from build123d import *

# Parameters (mm, degrees)
SKETCH1_W           = 82.6
SKETCH1_H           = 98
BOSS_EXTRUDE1_DEPTH = 1.2
SKETCH2_R           = 1.65
CUT_EXTRUDE1_DEPTH  = 129.172539961
SKETCH3_R           = 35
BOSS_EXTRUDE2_DEPTH = 8
SKETCH4_R           = 37
BOSS_EXTRUDE3_DEPTH = 1
SKETCH5_R           = 32
CUT_EXTRUDE2_DEPTH  = 129.572158728
CHAMFER1_SIZE       = 1


with BuildPart() as part:
    # Sketch1 → Boss-Extrude1 (new body)
    with BuildSketch(Plane.YZ):
        with Locations((41.3, 49)):
            Rectangle(SKETCH1_W, SKETCH1_H)
    extrude(amount=BOSS_EXTRUDE1_DEPTH)

    # Sketch2 → Cut-Extrude1 (cut, through all)
    with BuildSketch(Plane.YZ.offset(1.2)):
        with Locations(Location((3.2, 94.8, 0), (0, 0, 270))):
            Circle(SKETCH2_R)
        with Locations(Location((79.4, 94.8, 0), (0, 0, 270))):
            Circle(SKETCH2_R)
        with Locations(Location((3.2, 3.2, 0), (0, 0, 270))):
            Circle(SKETCH2_R)
        with Locations(Location((79.4, 3.2, 0), (0, 0, 270))):
            Circle(SKETCH2_R)
    extrude(amount=-CUT_EXTRUDE1_DEPTH, mode=Mode.SUBTRACT)

    # Sketch3 → Boss-Extrude2 (add)
    with BuildSketch(Plane.YZ.offset(1.2)):
        with Locations(Location((41.3, 49, 0), (0, 0, 270))):
            Circle(SKETCH3_R)
    extrude(amount=BOSS_EXTRUDE2_DEPTH)

    # Sketch4 → Boss-Extrude3 (add)
    with BuildSketch(Plane.YZ.offset(9.2)):
        with Locations(Location((41.3, 49, 0), (0, 0, 270))):
            Circle(SKETCH4_R)
    extrude(amount=BOSS_EXTRUDE3_DEPTH)

    # Sketch5 → Cut-Extrude2 (cut, through all)
    with BuildSketch(Plane.YZ.offset(10.2)):
        with Locations(Location((41.3, 49, 0), (0, 0, 270))):
            Circle(SKETCH5_R)
    extrude(amount=-CUT_EXTRUDE2_DEPTH, mode=Mode.SUBTRACT)

    # Chamfer1
    chamfer1_edges = [part.edges().sort_by_distance(p)[0] for p in [
        (0, 79.4, 96.45),
        (0, 3.2, 4.85),
        (0, 79.4, 4.85),
        (0, 3.2, 96.45),
        (0, 41.3, 81),
        (10.2, 41.3, 81),
    ]]
    chamfer(chamfer1_edges, length=CHAMFER1_SIZE)


solid = part.part
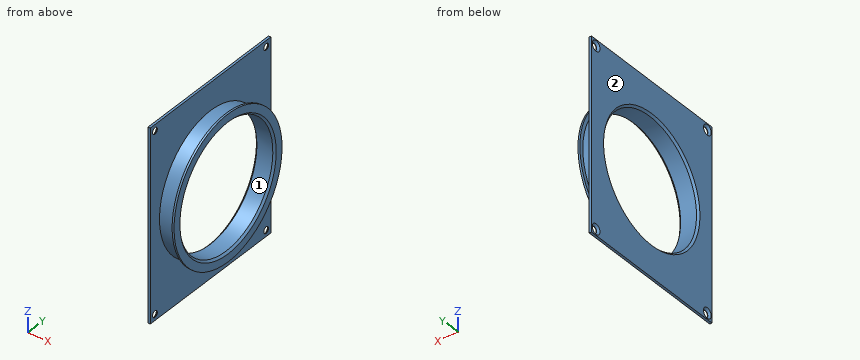
Source: CAD feature listing. Evaluate the final solid. Frame: model axes, mm. Face numbers are marked on the shaded views. Coordinates: 2 decimals unless noted, no trailing zeros. Loops run counter-clockwise (first coordinate to the right, second up) from the corner with the lowest first, then second, coordinate; pieces in that order, holes last. Notation, with made-up numbers: M -37,36.5 L 6,36.5 A19 cw 6,62.5 Z; hole C 8,67 d11. An arc over 180 degrees is marked long. Answer in a Markdown table with one row per item.
Q1. Section B-B on z = 94.8. Return the cut outline in (x, y).
Answers below:
| item | result |
|---|---|
| outline | M 0,0 L 1.2,0 L 1.2,1.55 L 1,1.55 L 0,0.55 Z; M 0,5.85 L 1,4.85 L 1.2,4.85 L 1.2,77.75 L 1,77.75 L 0,76.75 Z; M 0,82.05 L 1,81.05 L 1.2,81.05 L 1.2,82.6 L 0,82.6 Z |
Q2. Section D-D on z = 49. Return the cut outline in (x, y), plus the area to 3 significant figures.
Answers below:
| item | result |
|---|---|
| outline | M 0,0 L 1.2,0 L 1.2,6.3 L 9.2,6.3 L 9.2,4.3 L 10.2,4.3 L 10.2,8.3 L 9.2,9.3 L 1,9.3 L 0,8.3 Z; M 0,74.3 L 1,73.3 L 9.2,73.3 L 10.2,74.3 L 10.2,78.3 L 9.2,78.3 L 9.2,76.3 L 1.2,76.3 L 1.2,82.6 L 0,82.6 Z |
| area | 78.3 mm^2 |
Q3. First-contact query: pin 1 (5 mm diameter, centred on x = 7.5, y = 57, fed in from -Z); pin 2 (4 mm diameter, centred on y = 79.4, z = 94.8, fed in from +X); pin 3 (6 mm diameter, centred on x = 5, y = 46, fed in from +Z). Flat tips, straight axial feed; report the tip coordinate or a pass-through.
Answers below:
| item | result |
|---|---|
| pin 1 | stops at z = 14.7 |
| pin 2 | stops at x = 1.2 |
| pin 3 | stops at z = 83.96 |
Q4. Draft query along Z for the marked faces 1 and 2. Return one class per face: pulls with the +Z half, pulls with the -Z half, needs draft (parallel to the pull), parting line crosses it, or undercut.
Answers below:
| item | result |
|---|---|
| face 1 | undercut |
| face 2 | needs draft |
Q5. Section C-C on y = 41.3. Return the cut outline in (x, z).
Answers below:
| item | result |
|---|---|
| outline | M 0,0 L 1.2,0 L 1.2,14 L 9.2,14 L 9.2,12 L 10.2,12 L 10.2,16 L 9.2,17 L 1,17 L 0,16 Z; M 0,82 L 1,81 L 9.2,81 L 10.2,82 L 10.2,86 L 9.2,86 L 9.2,84 L 1.2,84 L 1.2,98 L 0,98 Z |
Q6. Section A-A on y = 3.2. Return the cut outline in (x, z).
Answers below:
| item | result |
|---|---|
| outline | M 0,0 L 1.2,0 L 1.2,1.55 L 1,1.55 L 0,0.55 Z; M 0,5.85 L 1,4.85 L 1.2,4.85 L 1.2,93.15 L 1,93.15 L 0,92.15 Z; M 0,97.45 L 1,96.45 L 1.2,96.45 L 1.2,98 L 0,98 Z |
Q7. Ray query, probe 1 along Z at (x, y) = (1.1, 79.4); probe 2 along Y at (x, z) = (1.15, 94.8); probe 3 along X at (y, z) = (49.5, 4.5). Return the intervals inside material, ascending. Write a range as from..to.
Answers below:
| item | result |
|---|---|
| probe 1 | z = 0..1.55, 4.85..93.15, 96.45..98 |
| probe 2 | y = 0..1.55, 4.85..77.75, 81.05..82.6 |
| probe 3 | x = 0..1.2 |
